For this review, use the dimensioned drawing (mm, ordinates from the lowest corner) and the shaded views. A direction names the side the tool comes from. Coordinates: 2 decimals unless noted, no trailing zeros. Loops run counter-clockwise (first coordinate to the right, second up) from the corner with the lowest first, then second, coordinate; pieces in that order, holes last.
1. To check wall thickness, follow probe 1 along Z at (x, y) = (3, 7.75); probe 2 along X at (y, z) = (5.5, 2.5); probe 3 along X at (y, z) = (3.25, 17) (1 decimal). State the ranges of each line that lie inside material, in increasing order.
2. Machinability: for the marked faces 1 and 2, which of the approach directions +Z, -Z, +X, -X, +Y, -Y give a long, thin tool a straight path to every point of the face, cutting with its end or side? Answer none if there is none.
3. Take a section at C-C, the plane x = 2.5. State the section outline as (y, z) points.
4. Take a section at A-A, the plane y = 4.75. State the section outline as (x, z) points (1 decimal).
5. Take a section at D-D, the plane y = 6.75. State the section outline as (x, z) points, then the cut area to 3 significant figures.
6. Clearance check with flat-ended pins moving along their axes: P1, Ø3, axis at x = 2, y = 5.5, coming from the -Z side; P2, Ø1.5, axis at x = 6, z = 5, coming from the +Y side. State where each tip first meets the part, or that it passes through.
7. Take a section at B-B, the plane z = 5. State the section outline as (x, y) points, then the cut area to 3 significant figures.
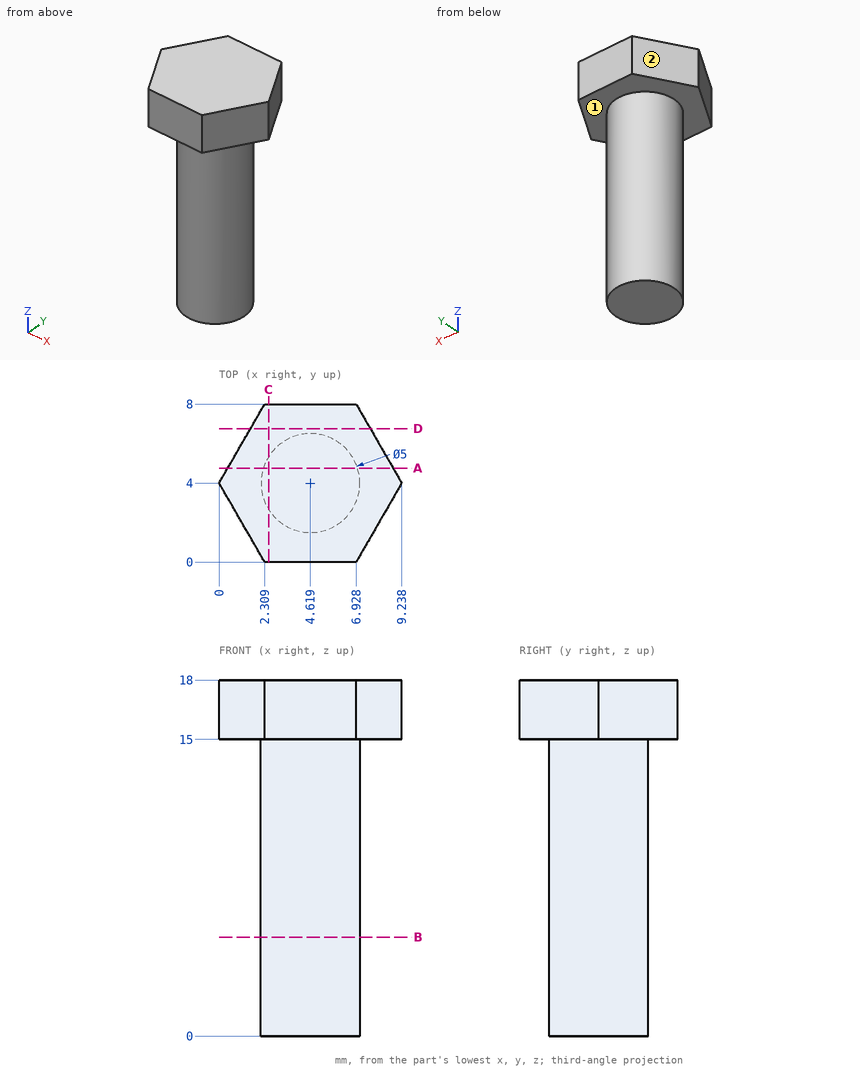
Results list:
1. probe 1: z = 15 to 18
1. probe 2: x = 2.62 to 6.62
1. probe 3: x = 0.4 to 8.8
2. face 1: -Z
2. face 2: +Z, -Z, -X, +Y
3. outline: (0, 15) - (2.67, 15) - (2.67, 0) - (5.33, 0) - (5.33, 15) - (8, 15) - (8, 18) - (0, 18) - close
4. outline: (0.4, 15) - (2.2, 15) - (2.2, 0) - (7, 0) - (7, 15) - (8.8, 15) - (8.8, 18) - (0.4, 18) - close
5. outline: (1.59, 15) - (7.65, 15) - (7.65, 18) - (1.59, 18) - close
5. area: 18.2 mm2
6. P1: stops at z = 0
6. P2: stops at y = 6.42
7. outline: circle Ø5 at (4.62, 4)
7. area: 19.6 mm2
